Read the model definition and answer for the solid it produces. Units are mm, in the model's axes. Coordinates: 2 decimals unless noted, no trailing zeros. Loops run counter-clockwise (first coordinate to the right, second up) from the corner with the lowest first, then second, coordinate; pieces in that order, holes last.
Q1. Section B-B (x = 39) is taken. Give the vertices of the cut face in (y, z).
Q2. Section C-C (z = 13.5) is taken. Give the vertices of the cut face in (x, y) (3 decimals), then the cut area to 3 significant figures.
Q3. Section A-A (y = 77.5) is taken. Give the vertices of the cut face in (x, z) (3 decimals), then the cut area to 3 significant figures.
Q4. Straight lines are drawn through the part: line 1 (X direction, y = 8, z = 12); line 2 (X direction, y = 42.5, z = 13.25) (3 decimals); line 3 (Z direction, x = 40.5, y = 96.5). For each, find the intervals that lie inside material, in ascending order.
Q5. Flat-ended cylindrical pins translate along their axes: P1, Ø1, axis at x = 38.5, y = 58.5, coming from the -Z side; P2, Ø2, axis at y = 62, z = 14.5, coming from the +X side (3 decimals); P3, Ø1.8, axis at x = 41.5, y = 62, coming from the +Z side. Find the tip coordinate at first contact, or state that the pin passes through.
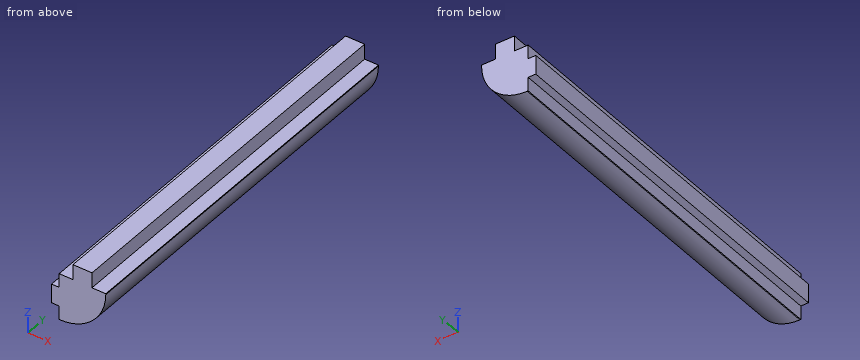
Autodesk Fusion 360 part; units mm, degrees
sketch "Sketch1" plane through (0, 0, 52.25) normal (0, 0, 1) x (-1, 0, 0)
  line L0 (12.25, -100) -> (12.25, 0)
  line L1 (12.25, 0) -> (0, 0)
  line L2 (0, 0) -> (0, -100)
  line L3 (0, -100) -> (12.25, -100)
  line L4 (0, 0) -> (12.25, 0) construction
  line L5 (6.125, 0) -> (8.625, 0) construction
  line L6 (6.125, 0) -> (3.625, 0) construction
  line L7 (3.625, 0) -> (8.625, 0) construction
  line L8 (3.625, 0) -> (8.625, 0)
  line L9 (8.625, 0) -> (8.625, -100)
  line L10 (8.625, -100) -> (3.625, -100)
  line L11 (3.625, -100) -> (3.625, 0)
  dimension "d3" = 5
sketch "Sketch2" plane through (0, 100, 0) normal (0, 1, 0) x (-1, 0, 0)
  line L0 (-4, 8.6) -> (-4, 3.6)
  line L1 (-4, 3.6) -> (8.5, 3.6)
  line L2 (8.5, 3.6) -> (8.5, 10.6)
  line L3 (8.5, 10.6) -> (3.5, 10.6)
  line L4 (3.5, 10.6) -> (3.5, 8.6)
  line L5 (3.5, 8.6) -> (-4, 8.6)
sketch "Sketch3" plane through (0, 100, 0) normal (0, 1, 0) x (-1, 0, 0)
  line L0 (-43.625, 52.25) -> (-43.625, 50.25)
  line L1 (-43.625, 50.25) -> (-48.625, 50.25)
  line L2 (-48.625, 50.25) -> (-48.625, 52.25)
  line L3 (-48.625, 52.25) -> (-52.25, 52.25)
  line L4 (-52.25, 52.25) -> (-52.25, 12.25)
  line L5 (-52.25, 12.25) -> (-48.625, 12.25)
  line L6 (-48.625, 12.25) -> (-48.625, 16.25)
  line L7 (-48.625, 16.25) -> (-43.625, 16.25)
  line L8 (-43.625, 16.25) -> (-43.625, 12.25)
  line L9 (-43.625, 12.25) -> (-40, 12.25)
  line L10 (-40, 12.25) -> (-40, 52.25)
  line L11 (-40, 52.25) -> (-43.625, 52.25)
  line L12 (-40, 0) -> (-56, 0) construction
  line L13 (-52.25, 12.25) -> (-48.625, 12.25)
  line L14 (-48.625, 16.25) -> (-48.625, 12.25)
  line L15 (-43.625, 16.25) -> (-48.625, 16.25)
  line L16 (-43.625, 12.25) -> (-43.625, 16.25)
  line L17 (-40, 12.25) -> (-43.625, 12.25)
  line L18 (-40, 8.6) -> (-40, 12.25)
  line L19 (-38, 8.6) -> (-40, 8.6)
  line L20 (-38, 3.6) -> (-38, 8.6)
  line L21 (-40, 3.6) -> (-38, 3.6)
  line L22 (-40, 0) -> (-40, 3.6)
  line L23 (-40, 0) -> (-52.25, 0)
  line L24 (-52.25, 12.25) -> (-52.25, 0)
extrude "Extrude3" add sketch "Sketch3" against normal blind 100 contours L5 L6 L7 L8 L9 L13 L14 L15 L16 L17 L18 L19 L20 L21 L22 L23 L24
fillet "Fillet1" radius 12 1 edges at (52.25, 50, 0)
Numbers:
1. outline: (0, 3.6) - (100, 3.6) - (100, 8.6) - (0, 8.6) - close
2. outline: (43.625, 0) - (48.625, 0) - (48.625, 100) - (43.625, 100) - close
2. area: 500 mm2
3. outline: (38, 3.6) - (40, 3.6) - (40, 0) - (40.25, 0) arc R12 ccw to (52.25, 12) - (52.25, 12.25) - (48.625, 12.25) - (48.625, 16.25) - (43.625, 16.25) - (43.625, 12.25) - (40, 12.25) - (40, 8.6) - (38, 8.6) - close
3. area: 149 mm2
4. line 1: x = 40 to 52.25
4. line 2: x = 43.625 to 48.625
4. line 3: z = 0 to 12.25
5. P1: stops at z = 3.6
5. P2: stops at x = 48.625
5. P3: stops at z = 12.25
